Autodesk Inventor part; units mm, degrees
ref_plane "YZ Plane" through (0, 0, 0) normal (1, 0, 0) x (0, 1, 0)
ref_plane "XZ Plane" through (0, 0, 0) normal (0, 1, 0) x (-1, 0, 0)
ref_plane "XY Plane" through (0, 0, 0) normal (0, 0, 1) x (1, 0, 0)
sketch "Sketch1" plane through (0, 0, 0) normal (0, 0, 1) x (1, 0, 0)
  line L0 (0, 0) -> (58.1152, 0)
  line L1 (58.1152, 0) -> (58.1152, 57.785)
  line L2 (58.1152, 57.785) -> (0, 57.785)
  line L3 (0, 57.785) -> (0, 0)
  line L4 (0, 43.4975) -> (58.1152, 43.4975)
  line L5 (0, 28.8925) -> (58.1152, 28.8925)
  line L6 (0, 14.2875) -> (58.1152, 14.2875)
  line L7 (29.0576, 57.785) -> (29.0576, 0)
  line L8 (16.3576, 57.785) -> (16.3576, 0)
  line L9 (41.7576, 57.785) -> (41.7576, 0)
  line L10 (1.2446, 43.4975) -> (1.2446, 14.2875)
  line L11 (56.8706, 43.4975) -> (56.8706, 14.2875)
  line L12 (16.3576, 56.7436) -> (41.7576, 56.7436)
  line L13 (16.3576, 1.0414) -> (41.7576, 1.0414)
  line L14 (4.9602, 57.785) -> (10.8826, 57.785) construction
  line L15 (0, 52.54) -> (5.245, 57.785)
  line L16 (58.1152, 52.54) -> (52.8702, 57.785)
  line L17 (0, 5.245) -> (5.245, 0)
  line L18 (58.1152, 5.245) -> (52.8702, 0)
  line L19 (41.7576, 56.242) -> (16.3576, 56.242)
  line L20 (41.7576, 1.543) -> (16.3576, 1.543)
  line L21 (41.7576, 57.785) -> (40.2146, 56.242)
  line L22 (16.3576, 57.785) -> (17.9006, 56.242)
  line L23 (41.7576, 0) -> (40.2146, 1.543)
  line L24 (16.3576, 0) -> (17.9006, 1.543)
  line L25 (37.6746, 57.785) -> (37.6746, 56.242)
  line L26 (20.4406, 57.785) -> (20.4406, 56.242)
  line L27 (37.6746, 0) -> (37.6746, 1.543)
  line L28 (20.4406, 0) -> (20.4406, 1.543)
  point P0 (52.8702, 0)
  point P1 (17.399, 1.0414)
  point P2 (40.7162, 1.0414)
  point P3 (17.399, 56.7436)
  point P4 (40.7162, 56.7436)
  point P5 (20.4406, 56.7436)
  point P6 (37.6746, 56.7436)
  point P7 (20.4406, 1.0414)
  point P8 (37.6746, 1.0414)
  dimension "d0" = 58.1152
  dimension "d1" = 57.785
  dimension "d2" = 29.21
  dimension "d3" = 25.4
  dimension "d4" = 55.626
  dimension "d5" = 55.7022
  dimension "d18" = 74.5363
  dimension "d19" = 45
  dimension "d34" = 54.6989
  dimension "d35" = 45
  dimension "d36" = 2.54
extrude "Extrusion1" add sketch "Sketch1" along normal blind 24.892
extrude "Extrusion2" cut sketch "Sketch1" along normal through all contours L24 L13 L28 L0 | L3 L5 L10 L6 | L28 L13 L7 L0 | L24 L20 L28 L13 | L3 L4 L10 L5 | L7 L13 L27 L0 | L27 L13 L23 L0 | L27 L20 L23 L13 | L2 L26 L12 L22 | L11 L5 L1 L6 | L2 L7 L12 L26 | L12 L26 L19 L22 | L11 L4 L1 L5 | L2 L25 L12 L7 | L25 L12 L21 L19 | L2 L21 L12 L25
extrude "Extrusion3" cut sketch "Sketch1" along normal through all contours L3 L17 L0 | L3 L2 L15 | L18 L1 L0 | L16 L2 L1
chamfer "Chamfer5" distance 3.175 angle 45 8 edges at (2.6225, 55.1625, 24.892) (55.4927, 55.1625, 24.892) (55.4927, 2.6225, 24.892) (2.6225, 2.6225, 24.892) (2.6225, 2.6225, 0) (2.6225, 55.1625, 0) (55.4927, 55.1625, 0) (55.4927, 2.6225, 0)
chamfer "Chamfer6" distance 3.175 angle 45 8 edges at (0, 45.7737, 0) (13.0464, 57.785, 0) (45.0688, 0, 0) (58.1152, 12.0113, 0) (0, 45.7737, 24.892) (13.0464, 57.785, 24.892) (58.1152, 12.0113, 24.892) (45.0688, 0, 24.892)
chamfer "Chamfer7" distance 0.5017 angle 45 4 edges at (37.6746, 56.7436, 12.446) (20.4406, 56.7436, 12.446) (37.6746, 1.0414, 12.446) (20.4406, 1.0414, 12.446)
chamfer "Chamfer8" distance 1.2446 angle 45 4 edges at (58.1152, 43.4975, 12.446) (58.1152, 14.2875, 12.446) (0, 43.4975, 12.446) (0, 14.2875, 12.446)
properties part number "Inclinometer" material "ABS Plastic"
The model under review builds one solid part; all positions refer to its coordinate system, in mm. A direction names the side the tool comes from. Coordinates: 2 decimals unless noted, no trailing zeros. Write each loop counter-clockwise with the first axis right and the second up, starting at its lowest first coordinate (ties: lowest second). Pieces come first, ordered by that corner, then holes. Notation, with made-up numbers: (41, 60.5) - (95, 60.5) arc R22 cw to (95, 82.5) - close; hole circle Ø11 at (78.25, 81). An arc over 180 degrees is marked (long way). Answer in a Markdown table with one row per item. Add a question column.
Q1. To check wall thickness, follow line 1 along X through (y, z) = (26, 10.25); line 2 along Y through (x, z) = (32, 10); line 3 along X through (y, z) = (5, 21) (3 decimals). State the ranges of each line that lie inside material, in increasing order. Write a range as from..to.
Q2. Clearance check with flat-ended pins moving along their axes: pin 1 (2 mm diameter, centred on x = 39.5, z = 14.5, fed in from -Y); pin 2 (6.5 mm diameter, centred on y = 31, z = 9.5, fed in from +X); pin 3 (3 mm diameter, centred on x = 39.5, z = 13.5, fed in from +Y). State where each tip first meets the part, or that it passes through.
Q3. Draft analysis for pull direction X (two halves, no side actions). For faces 1 (the face through (29, 1.041, 12)), 2 (the face through (3.797, 3.724, 23.327)), 3 (the face through (55.53, 2.66, 12.32)), state which applies: +X half, -X half, draft (parallel to the pull), parting line (faces both ways), or undercut.
Q4. Consider section B-B on x = 27. Give the boundary of the cut face in (y, z).
Q5. Consider section A-A on y = 21.5. Give the boundary of the cut face in (x, z).
Q6. For faces 4 (the face through (41, 0.76, 12.29)), 5 (the face through (19, 56.242, 12)), 6 (the face through (47, 0, 12)), list the 3-axis set-ups (+Z, -Z, +X, -X, +Y, -Y) from which the entire face can be reached by the end or side of a thin tool; tool diameter is ignored.
Answers below:
| question | item | result |
|---|---|---|
| 1 | line 1 | 1.24..56.87 |
| 1 | line 2 | 1.04..56.74 |
| 1 | line 3 | 0.245..57.87 |
| 2 | pin 1 | y = 1.26 |
| 2 | pin 2 | x = 56.87 |
| 2 | pin 3 | y = 57.03 |
| 3 | face 1 | undercut |
| 3 | face 2 | -X half |
| 3 | face 3 | +X half |
| 4 | outline | (1.04, 2.13) - (3.17, 0) - (54.61, 0) - (56.74, 2.13) - (56.74, 22.76) - (54.61, 24.89) - (3.17, 24.89) - (1.04, 22.76) - close |
| 5 | outline | (1.24, 1.93) - (3.17, 0) - (54.94, 0) - (56.87, 1.93) - (56.87, 22.96) - (54.94, 24.89) - (3.17, 24.89) - (1.24, 22.96) - close |
| 6 | face 4 | +Z, -Z, -Y |
| 6 | face 5 | +Z, -Z, +Y |
| 6 | face 6 | +Z, -Z, +X, -X, -Y |
